Autodesk Inventor part; units mm, degrees
ref_plane "Work Plane1" through (-23.745, -60.7506, 2.0147) normal (0, 0, 1) x (1, 0, 0)
ref_plane "YZ Plane" through (0, 0, 0) normal (1, 0, 0) x (0, 1, 0)
ref_plane "XZ Plane" through (0, 0, 0) normal (0, 1, 0) x (-1, 0, 0)
sketch "Sketch1" plane through (0, 0, 0) normal (0, 0, 1) x (1, 0, 0)
  circle A0 centre (13.604, -26.2353) radius 1.6
  line L0 (18.604, -44.1888) -> (15.604, -44.1888)
  line L1 (15.604, -44.1888) -> (15.604, -37.1888)
  line L2 (15.604, -37.1888) -> (18.604, -37.1888)
  line L3 (18.604, -26.2353) -> (18.604, -37.1888)
  arc A1 (18.604, -26.2353) -> (8.604, -26.2353) centre (13.604, -26.2353) ccw
  line L4 (8.604, -26.2353) -> (8.604, -45.6888)
  line L5 (9.104, -46.1888) -> (8.604, -45.6888)
  line L6 (9.104, -46.1888) -> (12.604, -46.1888)
  line L7 (13.104, -46.6888) -> (12.604, -46.1888)
  line L8 (13.104, -46.6888) -> (13.104, -55.1706)
  line L9 (12.604, -55.6706) -> (13.104, -55.1706)
  line L10 (12.604, -55.6706) -> (3.2048, -55.6706)
  line L11 (3.2048, -55.6706) -> (3.2048, -62.5334)
  line L12 (3.2048, -62.5334) -> (8.604, -62.5334)
  line L13 (8.604, -62.5334) -> (8.604, -81.1802)
  line L14 (8.604, -81.1802) -> (9.604, -81.1802)
  line L15 (9.604, -62.5334) -> (9.604, -81.1802)
  line L16 (9.604, -62.5334) -> (17.604, -62.5334)
  line L17 (17.604, -81.1802) -> (17.604, -62.5334)
  line L18 (17.604, -81.1802) -> (18.604, -81.1802)
  line L19 (18.604, -44.1888) -> (18.604, -81.1802)
  line L20 (19.104, -37.6888) -> (16.104, -37.6888)
  line L21 (16.104, -37.6888) -> (16.104, -43.6888)
  line L22 (16.104, -43.6888) -> (19.104, -43.6888)
  line L23 (19.104, -43.6888) -> (19.104, -81.6802)
  line L24 (19.104, -81.6802) -> (17.104, -81.6802)
  line L25 (17.104, -81.6802) -> (17.104, -63.0334)
  line L26 (17.104, -63.0334) -> (10.104, -63.0334)
  line L27 (10.104, -63.0334) -> (10.104, -81.6802)
  line L28 (10.104, -81.6802) -> (8.104, -81.6802)
  line L29 (8.104, -81.6802) -> (8.104, -63.0334)
  line L30 (8.104, -63.0334) -> (2.7048, -63.0334)
  line L31 (2.7048, -63.0334) -> (2.7048, -55.1706)
  line L32 (2.7048, -55.1706) -> (12.3969, -55.1706)
  line L33 (12.3969, -55.1706) -> (12.604, -54.9635)
  line L34 (12.604, -54.9635) -> (12.604, -46.8959)
  line L35 (12.604, -46.8959) -> (12.3969, -46.6888)
  line L36 (12.3969, -46.6888) -> (8.8969, -46.6888)
  line L37 (8.8969, -46.6888) -> (8.104, -45.8959)
  line L38 (8.104, -45.8959) -> (8.104, -26.2353)
  arc A2 (19.104, -26.2353) -> (8.104, -26.2353) centre (13.604, -26.2353) ccw
  line L39 (19.104, -26.2353) -> (19.104, -37.6888)
  line L40 (30.104, -37.6888) -> (30.104, -43.6888)
  line L41 (19.604, -38.1888) -> (16.604, -38.1888)
  line L42 (16.604, -38.1888) -> (16.604, -43.1888)
  line L43 (16.604, -43.1888) -> (19.604, -43.1888)
  line L44 (19.604, -43.1888) -> (19.604, -82.1802)
  line L45 (19.604, -82.1802) -> (16.604, -82.1802)
  line L46 (16.604, -82.1802) -> (16.604, -63.5334)
  line L47 (16.604, -63.5334) -> (10.604, -63.5334)
  line L48 (10.604, -63.5334) -> (10.604, -82.1802)
  line L49 (10.604, -82.1802) -> (7.604, -82.1802)
  line L50 (7.604, -82.1802) -> (7.604, -63.5334)
  line L51 (7.604, -63.5334) -> (2.2048, -63.5334)
  line L52 (2.2048, -63.5334) -> (2.2048, -54.6706)
  line L53 (2.2048, -54.6706) -> (12.104, -54.6706)
  line L54 (12.104, -54.6706) -> (12.104, -47.1888)
  line L55 (12.104, -47.1888) -> (8.6898, -47.1888)
  line L56 (8.6898, -47.1888) -> (7.604, -46.103)
  line L57 (7.604, -46.103) -> (7.604, -26.2353)
  arc A3 (19.604, -26.2353) -> (7.604, -26.2353) centre (13.604, -26.2353) ccw
  line L58 (19.604, -26.2353) -> (19.604, -38.1888)
  circle A4 centre (9.4965, -50.9297) radius 1.5
  line L59 (30.104, -37.6888) -> (35.104, -37.6888)
  line L60 (13.604, -20.7353) -> (35.104, -20.7353)
  line L61 (13.604, -20.7353) -> (35.104, -20.7353) construction
  line L62 (12.104, -54.6706) -> (35.104, -54.6706)
  line L63 (35.104, -54.6706) -> (35.104, -20.7353)
  line L64 (6.389, 0.2) -> (6.389, -55.4706)
  line L65 (19.604, -54.6706) -> (25.604, -54.6706)
  line L66 (35.104, -20.7353) -> (32.104, -20.7353)
  line L67 (32.104, -24.7353) -> (32.104, -52.4297)
  line L68 (9.4965, -50.9297) -> (32.104, -50.9297)
  circle A5 centre (32.104, -26.2353) radius 1.5
  circle A6 centre (32.104, -50.9297) radius 1.5
  line L69 (25.604, -54.6706) -> (23.3357, -43.6888)
  line L70 (16.104, -37.6888) -> (19.604, -37.6888)
  line L71 (22.0964, -37.6888) -> (30.104, -37.6888)
  line L72 (30.104, -43.6888) -> (23.3357, -43.6888)
  line L73 (19.604, -43.6888) -> (19.104, -43.6888)
  line L74 (22.0964, -37.6888) -> (19.4799, -25.0216)
  line L75 (18.5946, -20.7353) -> (18.0297, -18.0002)
  line L76 (13.604, -26.2353) -> (19.7306, -26.2353)
  line L77 (30.604, -26.2353) -> (32.104, -26.2353)
  point P0 (0, 0)
  point P1 (16.0019, -20.7353)
  dimension "d10" = 3
  dimension "d0" = 0.5
  dimension "d2" = 14
  dimension "d3" = 0.5
  dimension "d4" = 5
  dimension "d5" = 0
  dimension "d6" = 3.1842
  dimension "d7" = 6
  dimension "d8" = 3
  dimension "d9" = 3
extrude "Extrusion1" add sketch "Sketch1" along normal blind 7 contours L69 L72 L40 L59 L67 A6 L68 | L68 A6 L67 L59 L63 L62 L69 | L60 L63 L59 L71 L74 A3
sketch "Sketch2" plane through (0, 0, 7) normal (0, 0, 1) x (1, 0, 0)
  line L0 (25.604, -54.6706) -> (35.104, -54.6706)
  line L1 (35.104, -54.6706) -> (35.104, -20.7353)
  line L2 (35.104, -20.7353) -> (16.0019, -20.7353)
  arc A0 (19.4799, -25.0216) -> (16.0019, -20.7353) centre (13.604, -26.2353) ccw
  line L3 (19.4799, -25.0216) -> (22.0964, -37.6888)
  line L4 (22.0964, -37.6888) -> (30.104, -37.6888)
  line L5 (30.104, -37.6888) -> (30.104, -43.6888)
  line L6 (30.104, -43.6888) -> (23.3357, -43.6888)
  line L7 (23.3357, -43.6888) -> (25.604, -54.6706)
  circle A1 centre (32.104, -50.9297) radius 1.5
  circle A2 centre (32.104, -26.2353) radius 1.5
  circle A3 centre (13.604, -26.2353) radius 1.5
  circle A4 centre (9.4965, -50.9297) radius 1.5
  line L8 (6.389, 0.2) -> (6.389, -55.4706)
  line L9 (35.104, -20.7353) -> (6.389, -20.7353)
  line L10 (25.604, -54.6706) -> (35.104, -54.6706)
  line L11 (35.104, -54.6706) -> (6.389, -54.6706)
  point P0 (0, 0)
extrude "Extrusion2" add sketch "Sketch2" along normal blind 1.5
sketch "Sketch3" plane through (0, 0, 7) normal (0, 0, -1) x (-1, 0, 0)
  line L0 (-15.604, -37.1888) -> (-15.604, -44.1888)
  line L1 (-18.604, -37.1888) -> (-15.604, -37.1888)
  line L2 (-15.604, -44.1888) -> (-18.604, -44.1888)
  line L3 (-19.4799, -25.0216) -> (-22.0964, -37.6888)
  arc A0 (-16.0019, -20.7353) -> (-19.4799, -25.0216) centre (-13.604, -26.2353) ccw
  line L4 (-16.0019, -20.7353) -> (-6.389, -20.7353)
  line L5 (-6.389, -78.3802) -> (-6.389, 0.2)
  line L6 (-6.389, -54.6706) -> (-25.604, -54.6706)
  line L7 (-23.3357, -43.6888) -> (-25.604, -54.6706)
  line L8 (-15.604, -37.1888) -> (-21.9931, -37.1888)
  line L9 (-15.604, -44.1888) -> (-23.4389, -44.1888)
  circle A1 centre (-13.604, -26.2353) radius 1.5
  circle A2 centre (-9.4965, -50.9297) radius 1.5
  point P0 (0, 0)
extrude "Extrusion3" add sketch "Sketch3" along normal blind 4
sketch "Sketch4" plane through (0, 0, 8.5) normal (0, 0, 1) x (1, 0, 0)
  circle A0 centre (32.104, -26.2353) radius 1.5
  circle A1 centre (13.604, -26.2353) radius 1.5
  circle A2 centre (9.4965, -50.9297) radius 1.5
  circle A3 centre (32.104, -50.9297) radius 1.5
  circle A4 centre (32.104, -26.2353) radius 3.5
  circle A5 centre (13.604, -26.2353) radius 3.5
  circle A6 centre (32.104, -50.9297) radius 3.5
  circle A7 centre (9.4965, -50.9297) radius 3.5
  line L0 (35.104, -54.6706) -> (35.104, -20.7353)
  line L1 (6.389, -54.6706) -> (35.104, -54.6706)
  line L2 (6.5058, -78.3802) -> (6.5058, 0.2)
  line L3 (9.4965, -47.4297) -> (6.5058, -47.4297)
  line L4 (12.9965, -50.9297) -> (12.9965, -54.6706)
  line L5 (28.604, -50.9297) -> (28.604, -54.6706)
  line L6 (32.104, -47.4297) -> (35.104, -47.4297)
  line L7 (35.104, -29.7353) -> (32.104, -29.7353)
  line L8 (28.604, -26.2353) -> (28.604, -20.7353)
  line L9 (35.104, -20.7353) -> (16.0019, -20.7353)
  point P0 (0, 0)
  point P1 (6.5058, -54.6706)
  dimension "d17" = 7
  dimension "d18" = 7
  dimension "d19" = 7
  dimension "d20" = 7
extrude "Extrusion4" cut sketch "Sketch4" against normal blind 3 contours A4 L0 | L8 L9 L0 A4 | A4 L0 L7 | A5 | A6 L0 | L6 L0 A6 | A6 L0 L1 L5 | A7 L2 | L4 L1 L2 A7 | A7 L2 L3 picked at (34.604, -26.2353) picked at (34.604, -50.9297) picked at (7.0027, -50.9297)
sketch "Sketch5" plane through (0, 0, 8.5) normal (0, 0, 1) x (1, 0, 0)
  line L0 (6.5058, -54.6706) -> (6.5058, -47.4297)
  line L1 (6.389, -54.6706) -> (6.5058, -54.6706)
  line L2 (6.389, -20.7353) -> (6.389, -54.6706)
  line L3 (6.5058, -54.6706) -> (6.1522, -54.6706)
  line L4 (6.1522, -54.6706) -> (6.1522, -47.4297)
  line L5 (6.1522, -47.4297) -> (6.5058, -47.4297)
  line L6 (6.5058, -47.4297) -> (6.5058, -54.6706)
  point P0 (0, 0)
extrude "Extrusion5" cut sketch "Sketch5" against normal up to surface (3 mm away)
chamfer "Chamfer1" distance 2 angle 45 4 edges at (6.389, -34.0825, 8.5) (35.104, -38.5825, 8.5) (17.4965, -20.7353, 8.5) (20.8002, -54.6706, 8.5)
sketch "Sketch6" plane through (0, 0, 3) normal (0, 0, -1) x (-1, 0, 0)
  line L0 (-6.389, -54.6706) -> (-6.389, -20.7353)
  line L1 (-6.389, -55.1706) -> (-12.3969, -55.1706)
  line L2 (-12.604, -54.9635) -> (-12.3969, -55.1706)
  line L3 (-12.604, -46.8959) -> (-12.604, -54.9635)
  line L4 (-12.3969, -46.6888) -> (-12.604, -46.8959)
  line L5 (-8.404, -46.6888) -> (-12.3969, -46.6888)
  line L6 (-8.404, -20.7353) -> (-8.404, -46.6888)
  line L7 (-8.404, 3) -> (-8.404, -20.7353)
  line L8 (3.1786, 3) -> (-8.404, 3)
  line L9 (3.1786, 0.2) -> (3.1786, 3)
  line L10 (3.1786, 0.2) -> (-6.389, 0.2)
  line L11 (-6.389, 0.2) -> (-6.389, -55.1706)
  circle A0 centre (-9.4965, -50.9297) radius 1.5
  line L12 (-6.389, -20.7353) -> (-16.0019, -20.7353)
  line L13 (-25.604, -54.6706) -> (-6.389, -54.6706)
  point P0 (0, 0)
  point P1 (-12.604, -54.6706)
ref_plane "Work Plane1" through (-23.745, -60.7506, 2.0147) normal (0, 0, 1) x (1, 0, 0)
extrude "Extrusion6" add sketch "Sketch6" along normal up to surface (0.9853 mm away) contours L13 L3 L4 L5 L6 L12 L0
properties part number "LatchCover_3DPrint"
The listing builds one solid part. Answer for the finished solid, in the listing's coordinates (mm). A direction names the side the tool comes from. Round coordinates to 2 decimals unless told otherwise and drop trailing zeros. Order: outer loops, then holes, each group sorted by start corner. A loop starts at its lowest first (then second) coordinate and runs counter-clockwise, first axis right, second up. Notation, with made-up numbers: M -37.5,-30.75 L -30.5,-30.75 A13 cw -30.5,-5.75 Z; hole C 27.5,9.25 d3. An arc over 180 degrees is marked long. Answer in a Markdown table with one row per item. Add a question column.
1) The part is cut by section C-C on z = 4. Determine the outline of the cut face in (x, y).
2) Consider line 1 along Y through (x, z) = (28.5, 3.25); line 2 along Y through (x, z) = (15.75, 3.5); line 3 along Z through (x, y) = (30, -52). Determine where each line is inside the solid, lowest interval first. Write a range as from..to.
3) The part is cut by section D-D on y = -39. Determine the outline of the cut face in (x, z), plus the area to 3 significant figures.
4) Which of the six approach directions +Z, -Z, +X, -X, +Y, -Y give full straight-line access (tool end or side, diameter ignored) to faces 5 (the face through (33, -47.43, 7)), 6 (the face through (28.604, -24, 7)), 7 (the face through (10, -53, 5.5))?
5) Determine the mould class of faces 1 (the face through (19, -44.189, 5)), 2 (the face through (32, -24, 5.5)), 3 (the face through (14, -28, 5.5)), 4 (the face through (10.4, -46.689, 2.5)) for opening direction Y: pulls with the +Y half, pulls with the -Y half, needs draft (parallel to the pull), parting line crosses it, or undercut.
6) Flat-ended cylindrical pins translate along their axes: pin 1 Ø4 at (x, y) = (13.6, -26.24) entering from +Z; pin 2 Ø1.5 at (y, z) = (-53.5, 7) entering from -X; pin 3 Ø0.5 at (x, z) = (11.5, 2.5) entering from +Y. Find the tip coordinate at first contact, or state that the pin passes through.
7) The part is cut by section B-B on x = 14.5. Determine the outline of the cut face in (y, z).
8) The part is cut by section A-A on z = 1.25. Determine the outline of the cut face in (x, y).
Findings below:
| question | item | result |
|---|---|---|
| 1 | outline | M 6.39,-54.67 L 35.1,-54.67 L 35.1,-20.74 L 6.39,-20.74 Z; hole C 9.5,-50.93 d3; hole C 13.6,-26.24 d3; hole M 15.6,-44.19 L 23.44,-44.19 L 23.34,-43.69 L 30.1,-43.69 L 30.1,-37.69 L 22.1,-37.69 L 21.99,-37.19 L 15.6,-37.19 Z; hole C 32.1,-50.93 d3; hole C 32.1,-26.24 d3 |
| 2 | line 1 | y = -54.67..-43.69, -37.69..-20.74 |
| 2 | line 2 | y = -54.67..-44.19, -37.19..-20.74 |
| 2 | line 3 | z = 0..5.5 |
| 3 | outline | M 6.39,2.01 L 8.4,2.01 L 8.4,3 L 15.6,3 L 15.6,7 L 30.1,7 L 30.1,0 L 35.1,0 L 35.1,6.5 L 33.1,8.5 L 8.39,8.5 L 6.39,6.5 Z |
| 3 | area | 113 mm² |
| 4 | face 5 | +Z, +X, -Y |
| 4 | face 6 | +Z, +X, +Y |
| 4 | face 7 | +Z, -X, -Y |
| 5 | face 1 | undercut |
| 5 | face 2 | needs draft |
| 5 | face 3 | undercut |
| 5 | face 4 | pulls with the +Y half |
| 6 | pin 1 | stops at z = 5.5 |
| 6 | pin 2 | stops at x = 13 |
| 6 | pin 3 | stops at y = -46.69 |
| 7 | outline | M -54.67,3 L -27.44,3 L -27.44,5.5 L -29.62,5.5 L -29.62,8.5 L -52.67,8.5 L -54.67,6.5 Z; M -25.03,3 L -20.74,3 L -20.74,6.5 L -22.74,8.5 L -22.85,8.5 L -22.85,5.5 L -25.03,5.5 Z |
| 8 | outline | M 16,-20.74 A6 cw 19.48,-25.02 L 22.1,-37.69 L 30.1,-37.69 L 30.1,-43.69 L 23.34,-43.69 L 25.6,-54.67 L 35.1,-54.67 L 35.1,-20.74 Z; hole C 32.1,-50.93 d3; hole C 32.1,-26.24 d3 |
